CAD build for the part. Positions are in the model's coordinates, mm. A direction names the side the tool comes from. Coordinates: 2 decimals unless noted, no trailing zeros. Loops run counter-clockwise (first coordinate to the right, second up) from the corner with the lowest first, then second, coordinate; pieces in that order, holes last.
1) Saw through at A-A, the plane x = 0.5. Write the cut outline in (y, z), and give its area (3 significant figures).
2) Saw through at C-C, the plane z = 25.25. Write the cut outline in (x, y), and give its area (3 significant figures).
3) Wall check: line 1 along Z through (x, y) = (6.25, -8.25); line 2 along Y through (x, z) = (3, 23); line 3 along X through (y, z) = (-4.5, 8.75). Give the ranges that are in metal, low to high.
4) Two-plate mould, pull along Y, no slides. Class faces 1 (the cylindrical face through (6.58, -34.38, 13.8)), 2 (the flat face through (10, -25, 14)), 3 (the cylindrical face through (0.874, -1.141, 26.797)): +Y half, -Y half, draft (parallel to the pull), parting line (faces both ways), or undercut.
5) Saw through at D-D, the plane z = 6.5. Write the cut outline in (x, y).
6) Pin check, flat tips, straight feed: pin 1 Ø5 at (y, z) = (-26.25, 5.51) entering from -X; pin 2 Ø4 at (y, z) = (-27.5, 6.5) entering from +X; pin 3 Ø6.5 at (x, y) = (-5.5, -13.5) entering from -Z. Stop position of each tip, or through.
7) Which spindle directions (+Z, -Z, +X, -X, +Y, -Y) get a long thin tool onto all of the face, cutting with end or side? Do faces 4 (the flat face through (3, -24, 6)), 5 (the flat face through (5, -25, 0)), 6 (the flat face through (0, -16, 6)). Say none if no direction does.
8) Saw through at B-B, the plane y = -8.25. Write the cut outline in (x, z).
```python
from build123d import *

# Parameters (mm, degrees)
F1_DEPTH      = 50
F2_R          = 2
F3_DEPTH      = 25
F4_R          = 4.03
F5_DEPTH      = 28.8
F5_DEPTH_BACK = 25
F2_R_2        = 4.1
F6_DEPTH      = 7
F7_R          = 4


with BuildPart() as f1:
    # F0 (on Front) → F1 (new body)
    with BuildSketch(Plane.XZ):
        Polygon((0, 12), (0, 0), (10, 0), (10, 28), (-8, 28), (-8, 12), align=None)
    extrude(amount=F1_DEPTH)

    # F2 (on face) → F3 (cut)
    with BuildSketch(Plane.YZ.offset(10)):
        with Locations((-26.25, 5.513248)):
            Circle(F2_R)
        with Locations((-8.25, 5.4)):
            Circle(F2_R)
    extrude(amount=-F3_DEPTH, mode=Mode.SUBTRACT)

    # F4 (on Top) → F5 (cut, two sides)
    with BuildSketch(Plane.XY) as f5_sk:
        with Locations((2.73504, -35.590066)):
            Circle(F4_R)
    extrude(amount=F5_DEPTH, mode=Mode.SUBTRACT)
    extrude(f5_sk.sketch, amount=-F5_DEPTH_BACK, mode=Mode.SUBTRACT)

    # F2 (on face) → F6 (cut, symmetric)
    with BuildSketch(Plane.YZ.offset(10)):
        with Locations((-26.25, 5.513248)):
            Circle(F2_R_2)
        with Locations((-26.25, 5.513248)):
            Circle(F2_R, mode=Mode.SUBTRACT)
        with Locations((-8.25, 5.4)):
            Circle(F2_R_2)
        with Locations((-8.25, 5.4)):
            Circle(F2_R, mode=Mode.SUBTRACT)
    extrude(amount=F6_DEPTH, both=True, mode=Mode.SUBTRACT)

    # F7
    f7_edges = [f1.edges().sort_by_distance(p)[0] for p in [
        (1, -50, 28),
        (1, 0, 28),
        (10, -50, 14),
        (10, 0, 14),
    ]]
    fillet(f7_edges, radius=F7_R)


solid = f1.part
```
Data:
1. outline: (-50, 0) - (-38.94, 0) - (-38.94, 28) - (-46, 28) arc R4 ccw to (-50, 24) - close; (-32.24, 0) - (0, 0) - (0, 24) arc R4 ccw to (-4, 28) - (-32.24, 28) - close; hole circle Ø4 at (-26.25, 5.51); hole circle Ø4 at (-8.25, 5.4)
1. area: 1,180 mm2
2. outline: (-8, -49.8) - (7.25, -49.8) arc R4 ccw to (10, -46) - (10, -4) arc R4 ccw to (7.25, -0.2) - (-8, -0.2) - close; hole circle Ø8.06 at (2.74, -35.59)
2. area: 836 mm2
3. line 1: z = 0 to 1.3, 9.5 to 28
3. line 2: y = -50 to -39.61, -31.57 to 0
3. line 3: x = 0 to 10
4. face 1: undercut
4. face 2: draft
4. face 3: +Y half
5. outline: (0, -50) - (6, -50) arc R4 ccw to (10, -46) - (10, -30.23) - (3, -30.23) - (3, -27.99) - (0, -27.99) - (0, -32.63) arc R4.03 cw (long way) to (0, -38.55) - close; (0, -24.51) - (3, -24.51) - (3, -22.27) - (10, -22.27) - (10, -12.2) - (3, -12.2) - (3, -9.92) - (0, -9.92) - close; (0, -6.58) - (3, -6.58) - (3, -4.3) - (10, -4.3) - (10, -4) arc R4 ccw to (6, 0) - (0, 0) - close
6. pin 1: stops at x = 0
6. pin 2: stops at x = 3
6. pin 3: stops at z = 12
7. face 4: +X
7. face 5: -Z, +X, -X, +Y, -Y
7. face 6: -Z, -X, +Y, -Y
8. outline: (-8, 12) - (0, 12) - (0, 7.4) - (3, 7.4) - (3, 9.5) - (10, 9.5) - (10, 28) - (-8, 28) - close; (0, 0) - (10, 0) - (10, 1.3) - (3, 1.3) - (3, 3.4) - (0, 3.4) - close
